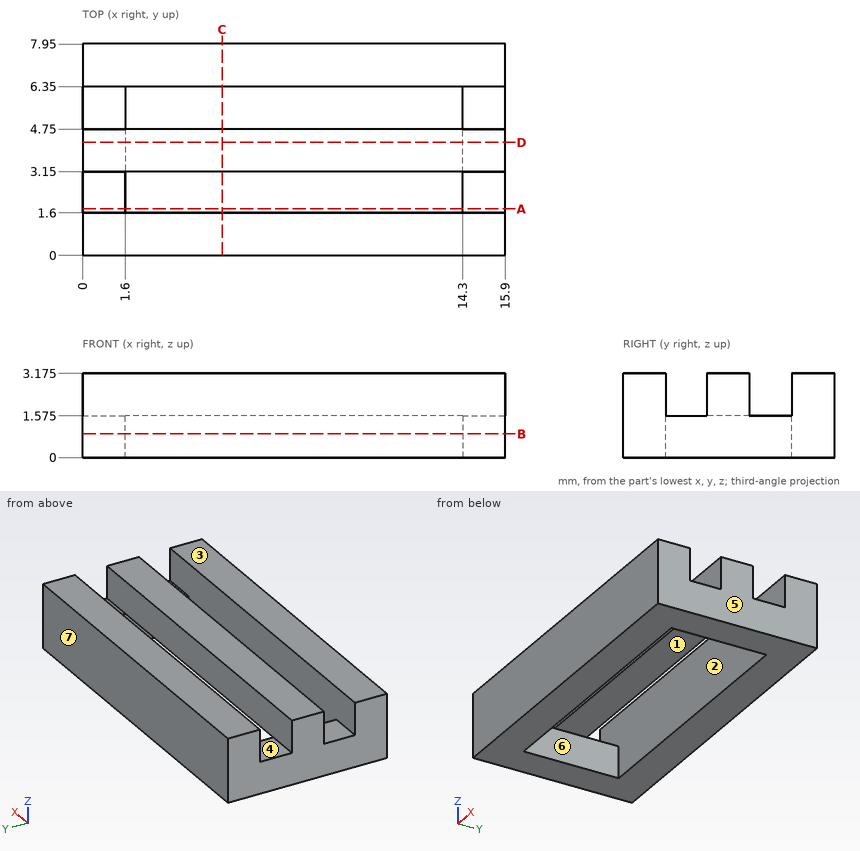
Geometry check sheet. Reference: drawing and pictorial views, mm from the part's lowest x, y, z. A direction names the side the tool comes from. Give positions to 0.01 mm unless a question says otherwise; leave off trailing zeros. Order: outer loops, then holes, each group sorted by start corner. A loop starts at its lowest first (then second) coordinate and runs counter-clockwise, first axis right, second up. Notation, with made-up numbers: M -34.5,10 L -27.5,10 A12 cw -27.5,24 Z; hole C -13,2 d7. An arc over 180 degrees is marked long. Answer in a Markdown table with one row per item. Add a question column.
Item 1: Gauge pin test, flat ends, axial feed: pin 1 (1.8 mm diameter, centred on x = 8.5, y = 4, fed in from -Z) (1 decimal); pin 2 (0.5 mm diameter, centred on x = 1, y = 6, fed in from +Z) (1 decimal). Record the tip position at first contact, or that the pin passes through.
Item 2: Section check D-D, the plane y = 4.25. Enter the section's corners in (x, z) (1 decimal), and give its area (3 significant figures).
Item 3: Mould release check, pull along X, two halves, no side actions. Record for the marked faces 5, 6 and 7: released by +X, released by -X, zero draft, split by the parting line, or undercut.
Item 4: Section check C-C, the plane x = 5.25. State how many separate pieces and enclosed holes the cut face has, and give its area (3 significant figures).
Item 5: Section check B-B, the plane z = 0.9. Enter the section's corners in (x, y).
Item 6: Scan lines: probe 1 along Y at (x, z) = (13.5, 2.1); probe 2 along Y at (x, z) = (2.5, 0.95). Record each from-to range of solid material in increasing order. Write a range as from..to.
Item 7: Tool access check on the marked faces 1, 2, 3 and 4. Record the directions out of +Z, -Z, +X, -X, +Y, -Y that give a thin tool (end or side, any length) a straight path to the whole face; none if there is none.
Item 8: Section check A-A, the plane y = 1.75. Enter the section's corners in (x, z) (1 decimal).
Filled sheet:
| question | item | result |
|---|---|---|
| 1 | pin 1 | stops at z = 1.6 |
| 1 | pin 2 | stops at z = 1.6 |
| 2 | outline | M 0,0 L 1.6,0 L 1.6,1.6 L 14.3,1.6 L 14.3,0 L 15.9,0 L 15.9,3.2 L 0,3.2 Z |
| 2 | area | 30.5 mm^2 |
| 3 | face 5 | released by +X |
| 3 | face 6 | undercut |
| 3 | face 7 | zero draft |
| 4 | separate pieces | 3 |
| 4 | enclosed holes | 0 |
| 4 | area | 12.7 mm^2 |
| 5 | outline | M 0,0 L 15.9,0 L 15.9,7.95 L 0,7.95 Z; hole M 1.6,1.6 L 14.3,1.6 L 14.3,6.35 L 1.6,6.35 Z |
| 6 | probe 1 | y = 0..1.6, 3.15..4.75, 6.35..7.95 |
| 6 | probe 2 | y = 0..1.6, 6.35..7.95 |
| 7 | face 1 | -Z |
| 7 | face 2 | +Z |
| 7 | face 3 | +Z, +X, -X, +Y, -Y |
| 7 | face 4 | +Z, +X, -X |
| 8 | outline | M 0,0 L 1.6,0 L 1.6,1.6 L 0,1.6 Z; M 14.3,0 L 15.9,0 L 15.9,1.6 L 14.3,1.6 Z |
